Autodesk Inventor part; units mm, degrees
ref_plane "a_XY" through (-12.7, 0, 0) normal (1, 0, 0) x (0, 0, -1)
ref_plane "a_YZ" through (-12.7, 0, 0) normal (0, 0, -1) x (0, 1, 0)
ref_plane "a_ZX" through (-12.7, 0, 0) normal (0, 1, 0) x (1, 0, 0)
sketch "Sketch_1" plane through (0, 0, 0) normal (0, 0, 1) x (1, 0, 0)
  line L0 (138.8872, 0) -> (0, 0)
  line L1 (0, 0) -> (0, 3.175)
  line L2 (0, 3.175) -> (138.8872, 3.175)
  line L3 (138.8872, 3.175) -> (138.8872, 0)
  line L4 (138.8872, 0) -> (0, 0)
revolve "Revolution1" add sketch "Sketch_1" angle 360 about axis through (138.8872, 0, 0) along (1, 0, 0)
sketch "Sketch_3" plane through (0, 0, 0) normal (0, 0, 1) x (1, 0, 0)
  line L0 (138.8872, 0) -> (116.713, 0)
  line L1 (116.713, 0) -> (116.713, 9.525)
  line L2 (116.713, 9.525) -> (138.8872, 9.525)
  line L3 (138.8872, 9.525) -> (138.8872, 0)
  line L4 (138.8872, 0) -> (116.713, 0)
revolve "Revolution2" add sketch "Sketch_3" angle 360 about axis through (138.8872, 0, 0) along (1, 0, 0)
sketch "Sketch_4" plane through (0, 0, 0) normal (0, 0, 1) x (1, 0, 0)
  line L0 (0, 0) -> (-12.7, 0)
  line L1 (-12.7, 0) -> (-12.7, 2.634)
  line L2 (-12.7, 2.634) -> (-12.159, 3.175)
  line L3 (-12.159, 3.175) -> (0, 3.175)
  line L4 (0, 3.175) -> (0, 0)
  line L5 (0, 0) -> (-12.7, 0)
revolve "Revolution3" add sketch "Sketch_4" angle 360 about axis through (0, 0, 0) along (1, 0, 0)
ref_plane "a_XY" through (-12.7, 0, 0) normal (1, 0, 0) x (0, 0, -1)
ref_plane "a_YZ" through (-12.7, 0, 0) normal (0, 0, -1) x (0, 1, 0)
ref_plane "a_ZX" through (-12.7, 0, 0) normal (0, 1, 0) x (1, 0, 0)
ref_plane "c1_XY" through (0, 0, 0) normal (1, 0, 0) x (0, 0, -1)
ref_plane "c1_YZ" through (0, 0, 0) normal (0, 0, -1) x (0, 1, 0)
ref_plane "c1_ZX" through (0, 0, 0) normal (0, 1, 0) x (1, 0, 0)
ref_plane "cc1_XY" through (0, 0, -3.175) normal (1, 0, 0) x (0, 0, -1)
ref_plane "cc1_YZ" through (0, 0, -3.175) normal (0, 0, -1) x (0, 1, 0)
ref_plane "cc1_ZX" through (0, 0, -3.175) normal (0, 1, 0) x (1, 0, 0)
ref_plane "cc2_XY" through (0, 0, 3.175) normal (1, 0, 0) x (0, 0, -1)
ref_plane "cc2_YZ" through (0, 0, 3.175) normal (0, 0, -1) x (0, 1, 0)
ref_plane "cc2_ZX" through (0, 0, 3.175) normal (0, 1, 0) x (1, 0, 0)
ref_plane "kk_XY" through (-6.35, 0, 3.175) normal (1, 0, 0) x (0, 0, -1)
ref_plane "kk_YZ" through (-6.35, 0, 3.175) normal (0, 0, -1) x (0, 1, 0)
ref_plane "kk_ZX" through (-6.35, 0, 3.175) normal (0, 1, 0) x (1, 0, 0)
ref_plane "rod_XY" through (138.8872, 0, 0) normal (1, 0, 0) x (0, 0, -1)
ref_plane "rod_YZ" through (138.8872, 0, 0) normal (0, 0, -1) x (0, 1, 0)
ref_plane "rod_ZX" through (138.8872, 0, 0) normal (0, 1, 0) x (1, 0, 0)
properties part number "5.4680.8730.50.500Double acting_00_005.4680.500.75N"
Can you work these out from the model? Positions are in its coordinate system, mm. A direction names the side the tool comes from. Coordinates: 2 decimals unless noted, no trailing zeros. Order: outer loops, then holes, each group sorted by start corner. A loop starts at its lowest first (then second) coordinate and runs counter-clockwise, first axis right, second up. Notation, with made-up numbers: (34, 69) - (77, 69) arc R34 cw to (77, 99) - close; hole circle Ø2 at (43.5, 34). An arc over 180 degrees is marked (long way). Answer in a Markdown table with one row per item.
1. Suppose I cut it at A-A (y = 0). Please give me the cut outline in (x, z) (3 decimals), and give its area (3 significant figures).
Reply:
| item | result |
|---|---|
| outline | (-12.7, -2.634) - (-12.159, -3.175) - (116.713, -3.175) - (116.713, -9.525) - (138.887, -9.525) - (138.887, 9.525) - (116.713, 9.525) - (116.713, 3.175) - (-12.159, 3.175) - (-12.7, 2.634) - close |
| area | 1,240 mm^2 |
2. Suppose I cut it at C-C (x = 67.5). Please give me the cut outline in (y, z) (3 decimals).
Reply:
| item | result |
|---|---|
| outline | circle Ø6.35 at (0, 0) |
3. If I drill on line 1 along X through (y, z) = (6.75, 1); line 2 along Y through (x, z) = (5, -1.75); line 3 along Z through (x, y) = (117, -2), over which ranges is the centre line in solid material (lowest first)?
Reply:
| item | result |
|---|---|
| line 1 | x = 116.71 to 138.89 |
| line 2 | y = -2.65 to 2.65 |
| line 3 | z = -9.31 to 9.31 |
4. Suppose I cut it at D-D (z = -5.75). Please give me the cut outline in (x, y), and give its area (3 significant figures).
Reply:
| item | result |
|---|---|
| outline | (116.71, -7.59) - (138.89, -7.59) - (138.89, 7.59) - (116.71, 7.59) - close |
| area | 337 mm^2 |
5. For pin 1 (6 mm diameter, centred on x = 54, y = 1, fed in from +Z) (3 decimals); pin 2 (1.5 mm diameter, centred on x = 96.5, z = 3, fed in from +Y); pin 3 (1.5 mm diameter, centred on x = 111, y = -1.5, fed in from +Z); pin 4 (3 mm diameter, centred on x = 43.5, y = 6.5, fed in from -Z), each with a flat end and sliding along its axis, tell me the tip position at first contact or that it passes through.
Reply:
| item | result |
|---|---|
| pin 1 | stops at z = 3.175 |
| pin 2 | stops at y = 2.24 |
| pin 3 | stops at z = 3.09 |
| pin 4 | passes through |
6. For faces 1 (the flat face through (-12.7, 0, 0)), 2 (the cylindrical face through (53.18, -0.69, -3.1)), which set-ups out of +Z, -Z, +X, -X, +Y, -Y let a thin tool reach every point of the face, with its end or its side?
Reply:
| item | result |
|---|---|
| face 1 | +Z, -Z, -X, +Y, -Y |
| face 2 | -X |
